```python
from build123d import *

# Parameters (mm, degrees)
F0_R     = 1.5
F1_DEPTH = 2
F2_R     = 3
F2_R_2   = 1.5
F3_DEPTH = 2
F7_DEPTH = 2


with BuildPart() as f1:
    # F0 (on Top) → F1 (new body)
    with BuildSketch(Plane.XY):
        with BuildLine():
            Line((97, 70), (3, 70))
            ThreePointArc((3, 70), (0.87868, 69.12132), (0, 67))
            Line((0, 67), (0, 3))
            ThreePointArc((0, 3), (0.87868, 0.87868), (3, 0))
            Line((3, 0), (97, 0))
            ThreePointArc((97, 0), (99.12132, 0.87868), (100, 3))
            Line((100, 3), (100, 4))
            Line((100, 4), (148, 4))
            ThreePointArc((148, 4), (150.12132, 4.87868), (151, 7))
            Line((151, 7), (151, 54))
            ThreePointArc((151, 54), (150.12132, 56.12132), (148, 57))
            Line((148, 57), (100, 57))
            Line((100, 57), (100, 67))
            ThreePointArc((100, 67), (99.12132, 69.12132), (97, 70))
        make_face()
        with Locations((9.65, 4.325)):
            Circle(F0_R, mode=Mode.SUBTRACT)
        with Locations((85.8, 4.325)):
            Circle(F0_R, mode=Mode.SUBTRACT)
        with Locations((9.65, 65.675)):
            Circle(F0_R, mode=Mode.SUBTRACT)
        with Locations((85.8, 65.675)):
            Circle(F0_R, mode=Mode.SUBTRACT)
    extrude(amount=-F1_DEPTH)

    # F2 (on face) → F3 (join)
    with BuildSketch(Plane(origin=(0, 0, -2), x_dir=(1, 0, 0), z_dir=(0, 0, -1))):
        with Locations((9.65, -65.675)):
            Circle(F2_R)
        with Locations((9.65, -65.675)):
            Circle(F2_R_2, mode=Mode.SUBTRACT)
        with Locations((85.8, -65.675)):
            Circle(F2_R)
        with Locations((85.8, -65.675)):
            Circle(F2_R_2, mode=Mode.SUBTRACT)
        with Locations((9.65, -4.325)):
            Circle(F2_R)
        with Locations((9.65, -4.325)):
            Circle(F2_R_2, mode=Mode.SUBTRACT)
        with Locations((85.8, -4.325)):
            Circle(F2_R)
        with Locations((85.8, -4.325)):
            Circle(F2_R_2, mode=Mode.SUBTRACT)
    extrude(amount=-F3_DEPTH)

    # F6 (on Top) → F7 (cut)
    with BuildSketch(Plane.XY):
        Polygon((34.263368, 12.735125), (72.459799, 12.735125), (106.358428, 32.306507), (22.963825, 32.306507), align=None)
        Polygon((106.358428, 37.693493), (72.459799, 57.264875), (34.263368, 57.264875), (22.963825, 37.693493), align=None)
        Polygon((94.823405, 8), (132.928523, 30), (112.928523, 30), (74.823405, 8), align=None)
        Polygon((112.928523, 40), (132.928523, 40), (94.823405, 62), (74.823405, 62), align=None)
    extrude(amount=-F7_DEPTH, mode=Mode.SUBTRACT)


solid = f1.part
```
Geometry check sheet. Reference: the model listing, model coordinates, mm. A direction names the side the tool comes from. Round coordinates to 2 decimals unless told otherwise and drop trailing zeros. Loops run counter-clockwise (first coordinate to the right, second up) from the corner with the lowest first, then second, coordinate; pieces in that order, holes last. Notation, with made-up numbers: (-24, 27.25) -> (7, 27.25) arc R32 ccw to (7, 55.25) -> close; hole circle Ø8 at (-28.75, 44). An arc over 180 degrees is marked (long way). Use a Markdown table: item, result.
(1) Set-up check for faces 5 (the cylindrical face through (99.1, 0.86, -0.99)), 6 (the flat face through (89.65, 47.34, -0.99)): record each of +Z, -Z, +X, -X, +Y, -Y from which the full face is reachable in a straight line by a thin tool's end or side.
Calculated:
| item | result |
|---|---|
| face 5 | +Z, -Z, +X, -Y |
| face 6 | +Z, -Z |
(2) Sectioned sample at C-C (y = 25). Enter the section's corners in (x, z), then the cut area to 3 significant figures.
Calculated:
| item | result |
|---|---|
| outline | (0, -2) -> (27.18, -2) -> (27.18, 0) -> (0, 0) -> close; (93.7, -2) -> (104.27, -2) -> (104.27, 0) -> (93.7, 0) -> close; (124.27, -2) -> (151, -2) -> (151, 0) -> (124.27, 0) -> close |
| area | 129 mm² |
(3) Scan lines: probe 1 along Y at (x, z) = (55.5, -1.55); probe 2 along Y at (x, z) = (9.65, -0.9) (3 decimals); probe 3 along X at (y, z) = (19.5, -0.25). Record each from-to range of solid material in increasing order.
Calculated:
| item | result |
|---|---|
| probe 1 | 0 to 12.74, 32.31 to 37.69, 57.26 to 70 |
| probe 2 | 0 to 2.825, 5.825 to 64.175, 67.175 to 70 |
| probe 3 | 0 to 30.36, 84.18 to 94.74, 114.74 to 151 |
(4) Mould release check, pull along X, two halves, no side actions. Record for faces 1 (the flat face through (74, 35, 0)), 2 (the flat face through (28.534, 22.658, -0.986)), 3 (the flat face through (89.2, 22.4, -1)), 4 (the cylindrical face through (150.1, 4.86, -0.99)): released by +X, released by -X, zero draft, split by the parting line, or undercut.
Calculated:
| item | result |
|---|---|
| face 1 | zero draft |
| face 2 | undercut |
| face 3 | undercut |
| face 4 | released by +X |
(5) Sectioned sample at D-D (x = 90). Enter the section's corners in (y, z).
Calculated:
| item | result |
|---|---|
| outline | (0, -2) -> (8, -2) -> (8, 0) -> (0, 0) -> close; (16.76, -2) -> (22.86, -2) -> (22.86, 0) -> (16.76, 0) -> close; (32.31, -2) -> (37.69, -2) -> (37.69, 0) -> (32.31, 0) -> close; (47.14, -2) -> (53.24, -2) -> (53.24, 0) -> (47.14, 0) -> close; (62, -2) -> (70, -2) -> (70, 0) -> (62, 0) -> close |
(6) Go/stop test with flat-tipped pins: P1, Ø0.6, axis at x = 136, z = -1, coming from the +Y side; P2, Ø1, axis at y = 63, z = -1.5, coming from the +X side; P3, Ø1, axis at x = 112.5, z = -1.5, coming from the -Y side. Record where each tip stops, or that it passes through.
Calculated:
| item | result |
|---|---|
| P1 | y = 57 |
| P2 | x = 100 |
| P3 | y = 4 |
(7) Sectioned sample at B-B (y = 11). Enter the section's corners in (x, z).
Calculated:
| item | result |
|---|---|
| outline | (0, -2) -> (80.02, -2) -> (80.02, 0) -> (0, 0) -> close; (100.02, -2) -> (151, -2) -> (151, 0) -> (100.02, 0) -> close |
(8) Sectioned sample at A-A (x = 9.65). Enter the section's corners in (y, z) (3 decimals), then the cut area to 3 significant figures.
Calculated:
| item | result |
|---|---|
| outline | (0, -2) -> (2.825, -2) -> (2.825, 0) -> (0, 0) -> close; (5.825, -2) -> (64.175, -2) -> (64.175, 0) -> (5.825, 0) -> close; (67.175, -2) -> (70, -2) -> (70, 0) -> (67.175, 0) -> close |
| area | 128 mm² |
